```python
from build123d import *

# Parameters (mm, degrees)
CROQUIS1_R              = 45
CROQUIS1_R_2            = 5
SALIENTE_EXTRUIR1_DEPTH = 30
SALIENTE_EXTRUIR2_START = -10
CROQUIS2_R              = 60
CROQUIS2_R_2            = 45
SALIENTE_EXTRUIR2_DEPTH = 10


with BuildPart() as part:
    # Croquis1 → Saliente-Extruir1 (new body)
    with BuildSketch(Plane(origin=(0, 0, 0), x_dir=(1, 0, 0), z_dir=(0, 1, 0))):
        Circle(CROQUIS1_R)
        Circle(CROQUIS1_R_2, mode=Mode.SUBTRACT)
        with Locations((0, 25)):
            Circle(CROQUIS1_R_2, mode=Mode.SUBTRACT)
        with Locations((25, 0)):
            Circle(CROQUIS1_R_2, mode=Mode.SUBTRACT)
        with Locations((0, -25)):
            Circle(CROQUIS1_R_2, mode=Mode.SUBTRACT)
        with Locations((-25, 0)):
            Circle(CROQUIS1_R_2, mode=Mode.SUBTRACT)
    extrude(amount=SALIENTE_EXTRUIR1_DEPTH)

    # Croquis2 → Saliente-Extruir2 (add)
    with BuildSketch(Plane(origin=(0, 30, 0), x_dir=(1, 0, 0), z_dir=(0, 1, 0)).offset(SALIENTE_EXTRUIR2_START)):
        Circle(CROQUIS2_R)
        Circle(CROQUIS2_R_2, mode=Mode.SUBTRACT)
    extrude(amount=-SALIENTE_EXTRUIR2_DEPTH)


solid = part.part
```
Could you check a few things on this model? Use its own coordinates, in mm. A direction names the side the tool comes from. Round coordinates to 2 decimals unless told otherwise and drop trailing zeros. Write each loop counter-clockwise with the first axis right and the second up, starting at its lowest first coordinate (ties: lowest second). Pieces come first, ordered by that corner, then holes. Notation, with made-up numbers: M -39,-31.5 L -15,-31.5 A19 cw -15,-9.5 Z; hole C 36.5,-1.75 d6. An arc over 180 degrees is marked long. Write each question's results on one line, items separated by ' | '. Start each with the question number.
1. Imagine slicing it at D-D on x = 25. List the corners of the cut face in (y, z) for me.
2. I'm going to push flat-ended pins straight in: pin 1 Ø4 at (y, z) = (18.5, 24) entering from -X; pin 2 Ø13 at (x, z) = (0, 0) entering from -Y; pin 3 Ø1 at (x, y) = (10.5, 25) entering from +Z; pin 4 Ø6 at (x, z) = (23.5, -44) entering from -Y. Where does each tip first touch, or does it pass through?
3. On a 3-axis mill with a long thin cutter (end or side, diameter ignored), from which of +Z, -Z, +X, -X, +Y, -Y can I reach the whole of each face in a straight line? I mean faces 1 (the face through (9, 0, -1)), 2 (the face through (20.765, 4.93, 39.923)), 3 (the face through (9, 20, -45)). Say none if no direction works.
4. Imagine slicing it at C-C on y = 16.25. List the corners of the cut face in (x, z) for me, and give its area (3 significant figures).
5. Thinking about a two-plate mould opening in Z: for faces 4 (the face through (20.765, 24.93, 39.923)), 5 (the face through (9, 10, -45)), 6 (the face through (20, 15, 0)), which applies, +Z half, -Z half, draft (parallel to the pull), parting line (faces both ways), or undercut?
6. I need wall thicknesses on L1, parallel to Z at x = 0, y = 16.25; L2, parallel to X at y = 21, z = 0. Which ranges of each line are inside material? Lowest first, please. Write a range as from..to.
7. Imagine slicing it at B-B on z = 0. List the corners of the cut face in (x, y) for me, and give its area (3 significant figures).
8. Imagine slicing it at A-A on x = 0. List the corners of the cut face in (y, z) for me, and give its area (3 significant figures).
Result sheet:
1) outline: M 0,-37.42 L 10,-37.42 L 10,-54.54 L 20,-54.54 L 20,-37.42 L 30,-37.42 L 30,-5 L 0,-5 Z; M 0,5 L 30,5 L 30,37.42 L 20,37.42 L 20,54.54 L 10,54.54 L 10,37.42 L 0,37.42 Z
2) pin 1: stops at x = -55.82 | pin 2: stops at y = 0 | pin 3: stops at z = 43.87 | pin 4: stops at y = 10
3) face 1: +Z, -Z, +X, -X, -Y | face 2: -Y | face 3: +Y
4) outline: C 0,0 d120; hole C -25,0 d10; hole C 0,-25 d10; hole C 0,0 d10; hole C 0,25 d10; hole C 25,0 d10 | area: 10,900 mm^2
5) face 4: parting line | face 5: draft | face 6: undercut
6) L1: z = -60..-30, -20..-5, 5..20, 30..60 | L2: x = -45..-30, -20..-5, 5..20, 30..45
7) outline: M -60,10 L -45,10 L -45,0 L -30,0 L -30,30 L -45,30 L -45,20 L -60,20 Z; M -20,0 L -5,0 L -5,30 L -20,30 Z; M 5,0 L 20,0 L 20,30 L 5,30 Z; M 30,0 L 45,0 L 45,10 L 60,10 L 60,20 L 45,20 L 45,30 L 30,30 Z | area: 2,100 mm^2
8) outline: M 0,-45 L 10,-45 L 10,-60 L 20,-60 L 20,-45 L 30,-45 L 30,-30 L 0,-30 Z; M 0,-20 L 30,-20 L 30,-5 L 0,-5 Z; M 0,5 L 30,5 L 30,20 L 0,20 Z; M 0,30 L 30,30 L 30,45 L 20,45 L 20,60 L 10,60 L 10,45 L 0,45 Z | area: 2,100 mm^2
